Read the model definition and answer for the solid it produces. Units are mm, in the model's axes. Face numbers are marked on the shaded views. Coordinates: 2 decimals unless noted, no trailing zeros. Write each loop counter-clockwise with the first axis right and the second up, starting at its lowest first coordinate (ties: lowest second). Pieces come first, ordered by that corner, then holes.
1) The part is cut by section A-A (x = 0). Determine the outline of the cut face in (y, z).
2) Find the intervals of material crossed by line 1 (Y direction, x = 0, z = 11.25); line 2 (Z direction, x = 11.5, y = 12.5); line 3 (Y direction, x = 18.5, z = 7), in increasing order.
3) Determine the mould class of the marked faces 1, 2 and 3 for opening direction X: +X half, -X half, draft (parallel to the pull), parting line (faces both ways), or undercut.
4) Each of these flat-tipped pins is pushed along its axis until it touches: pin 1 Ø12.5 at (x, y) = (-4, -2.5) entering from -Z; pin 2 Ø1 at (x, z) = (-17.5, 4) entering from +Y; pin 3 Ø1 at (y, z) = (19.5, 14.5) entering from +X; pin 4 Ø12 at (y, z) = (5.5, 3.5) entering from -X. Where does it stop, or does it pass through?
5) The part is cut by section C-C (z = 13). Determine the outline of the cut face in (x, y), then the cut area to 3 significant figures.
from build123d import *

# Parameters (mm, degrees)
F0_R     = 28.1156832237
F1_DEPTH = 25.4
F2_T     = -2.54
F3_R     = 5.08


with BuildPart() as f1:
    # F0 (on Top) → F1 (new body)
    with BuildSketch(Plane.XY):
        Circle(F0_R)
    extrude(amount=F1_DEPTH)

    # F2
    f2_openings = [f1.faces().sort_by_distance(p)[0] for p in [
        (0, 0, 0),
    ]]
    offset(amount=F2_T, openings=f2_openings)

    # F3
    f3_edges = [f1.edges().sort_by_distance(p)[0] for p in [
        (-25.575683, 0, 22.86),
    ]]
    fillet(f3_edges, radius=F3_R)


solid = f1.part
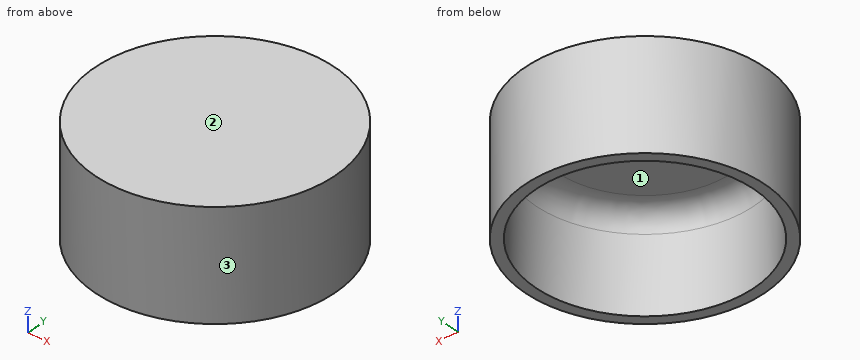
Reported:
1. outline: (-28.12, 0) - (-25.58, 0) - (-25.58, 17.78) arc R5.08 cw to (-20.5, 22.86) - (20.5, 22.86) arc R5.08 cw to (25.58, 17.78) - (25.58, 0) - (28.12, 0) - (28.12, 25.4) - (-28.12, 25.4) - close
2. line 1: y = -28.12 to -25.58, 25.58 to 28.12
2. line 2: z = 22.86 to 25.4
2. line 3: y = -21.17 to -17.66, 17.66 to 21.17
3. face 1: undercut
3. face 2: draft
3. face 3: parting line
4. pin 1: stops at z = 22.86
4. pin 2: stops at y = 22.39
4. pin 3: stops at x = 20.72
4. pin 4: stops at x = -28.12
5. outline: circle Ø56.23 at (0, 0); hole circle Ø51.15 at (0, 0)
5. area: 428 mm2
